Check sheet for the modelled part. Datum: model origin and axes. Units: mm. A direction names the side the tool comes from. Coordinates: 2 decimals unless noted, no trailing zeros. Loops run counter-clockwise (first coordinate to the right, second up) from the corner with the lowest first, then second, coordinate; pieces in that order, holes last.
```python
from build123d import *

# Parameters (mm, degrees)
F0_R     = 5
F1_DEPTH = 12.5
F2_DEPTH = 5
F3_R     = 5
F5_DEPTH = 7.5


with BuildPart() as f1:
    # F0 (on Front) → F1 (new body, symmetric)
    with BuildSketch(Plane.XZ):
        with BuildLine():
            ThreePointArc((6.8596340788, 11.9264922445), (6.9377952197, 12.139972805), (7.0173413473, 12.3529411765))
            ThreePointArc((7.0173413473, 12.3529411765), (6.8474920043, 11.9402854297), (6.6534014969, 11.5384615385))
            ThreePointArc((6.6534014969, 11.5384615385), (6.7556652076, 11.7329300253), (6.8596340788, 11.9264922445))
        make_face()
        with BuildLine():
            ThreePointArc((7.0173413473, -12.3529411765), (6.9377952197, -12.139972805), (6.8596340788, -11.9264922445))
            ThreePointArc((6.8596340788, -11.9264922445), (6.7556652076, -11.7329300253), (6.6534014969, -11.5384615385))
            ThreePointArc((6.6534014969, -11.5384615385), (6.8474920043, -11.9402854297), (7.0173413473, -12.3529411765))
        make_face()
        with BuildLine():
            ThreePointArc((6.6534014969, -11.5384615385), (-3.0597145703, -8.1525079957), (-7.0173413473, -17.6470588235))
            ThreePointArc((-7.0173413473, -17.6470588235), (-6.8474920043, -18.0597145703), (-6.6534014969, -18.4615384615))
            ThreePointArc((-6.6534014969, -18.4615384615), (1.7817812398, -22.2852766326), (7.5, -15))
            ThreePointArc((7.5, -15), (7.3783487348, -13.6546487642), (7.0173413473, -12.3529411765))
            ThreePointArc((7.0173413473, -12.3529411765), (6.8474920043, -11.9402854297), (6.6534014969, -11.5384615385))
        make_face()
        with Locations((0, -15)):
            Circle(F0_R, mode=Mode.SUBTRACT)
        with BuildLine():
            ThreePointArc((6.6534014969, 11.5384615385), (-3.0597145703, 8.1525079957), (-7.0173413473, 17.6470588235))
            ThreePointArc((-7.0173413473, 17.6470588235), (-10.2350656985, 0), (-7.0173413473, -17.6470588235))
            ThreePointArc((-7.0173413473, -17.6470588235), (-3.0597145703, -8.1525079957), (6.6534014969, -11.5384615385))
            ThreePointArc((6.6534014969, -11.5384615385), (6.7556652076, -11.7329300253), (6.8596340788, -11.9264922445))
            ThreePointArc((6.8596340788, -11.9264922445), (4.7649343015, 0), (6.8596340788, 11.9264922445))
            ThreePointArc((6.8596340788, 11.9264922445), (6.7556652076, 11.7329300253), (6.6534014969, 11.5384615385))
        make_face()
        with BuildLine():
            ThreePointArc((7.0173413473, 12.3529411765), (7.3783487348, 13.6546487642), (7.5, 15))
            ThreePointArc((7.5, 15), (1.7817812398, 22.2852766326), (-6.6534014969, 18.4615384615))
            ThreePointArc((-6.6534014969, 18.4615384615), (-6.8474920043, 18.0597145703), (-7.0173413473, 17.6470588235))
            ThreePointArc((-7.0173413473, 17.6470588235), (-3.0597145703, 8.1525079957), (6.6534014969, 11.5384615385))
            ThreePointArc((6.6534014969, 11.5384615385), (6.8474920043, 11.9402854297), (7.0173413473, 12.3529411765))
        make_face()
        with Locations((0, 15)):
            Circle(F0_R, mode=Mode.SUBTRACT)
    extrude(amount=F1_DEPTH, both=True)

    # F0 (on Front) → F2 (join, symmetric)
    with BuildSketch(Plane.XZ):
        with BuildLine():
            ThreePointArc((28.8314064867, -25), (16.0478683636, -21.4844397892), (6.8596340788, -11.9264922445))
            ThreePointArc((6.8596340788, -11.9264922445), (6.9377952197, -12.139972805), (7.0173413473, -12.3529411765))
            ThreePointArc((7.0173413473, -12.3529411765), (7.3783487348, -13.6546487642), (7.5, -15))
            ThreePointArc((7.5, -15), (1.7817812398, -22.2852766326), (-6.6534014969, -18.4615384615))
            ThreePointArc((-6.6534014969, -18.4615384615), (12.7660784434, -36.6320247169), (39.2872644776, -38.6092609833))
            Line((39.2872644776, -38.6092609833), (60, -33))
            Line((60, -33), (48.5096588292, -25))
            Line((48.5096588292, -25), (28.8314064867, -25))
        make_face()
        with BuildLine():
            ThreePointArc((37.2661231393, -28.311901738), (39.719379088, -29.7195718876), (38.3117089384, -32.1728278363))
            Line((38.3117089384, -32.1728278363), (23.8332360697, -36.0937745829))
            ThreePointArc((23.8332360697, -36.0937745829), (21.3799801209, -34.6861044333), (22.7876502706, -32.2328484846))
            Line((22.7876502706, -32.2328484846), (37.2661231393, -28.311901738))
        make_face(mode=Mode.SUBTRACT)
        with BuildLine():
            ThreePointArc((-6.6534014969, 18.4615384615), (1.7817812398, 22.2852766326), (7.5, 15))
            ThreePointArc((7.5, 15), (7.3783487348, 13.6546487642), (7.0173413473, 12.3529411765))
            ThreePointArc((7.0173413473, 12.3529411765), (6.9377952197, 12.139972805), (6.8596340788, 11.9264922445))
            ThreePointArc((6.8596340788, 11.9264922445), (16.0478683636, 21.4844397892), (28.8314064867, 25))
            Line((28.8314064867, 25), (48.5096588292, 25))
            Line((48.5096588292, 25), (60, 33))
            Line((60, 33), (39.2872644776, 38.6092609833))
            ThreePointArc((39.2872644776, 38.6092609833), (12.7660784434, 36.6320247169), (-6.6534014969, 18.4615384615))
        make_face()
        with BuildLine():
            ThreePointArc((22.7876502706, 32.2328484846), (21.3799801209, 34.6861044333), (23.8332360697, 36.0937745829))
            Line((23.8332360697, 36.0937745829), (38.3117089384, 32.1728278363))
            ThreePointArc((38.3117089384, 32.1728278363), (39.719379088, 29.7195718876), (37.2661231393, 28.311901738))
            Line((37.2661231393, 28.311901738), (22.7876502706, 32.2328484846))
        make_face(mode=Mode.SUBTRACT)
    extrude(amount=F2_DEPTH, both=True)

    # F3 (on face) → F5 (cut, symmetric)
    with BuildSketch(Plane(origin=(0, 12.5, 0), x_dir=(-1, 0, 0), z_dir=(0, 1, 0))):
        with Locations((2.7350656985, 0)):
            Circle(F3_R)
    extrude(amount=F5_DEPTH, both=True, mode=Mode.SUBTRACT)


solid = f1.part
```
1) Section check B-B on z = 0. Enter the section's corners in (x, y), plus the area to 3 significant figures.
Answer sheet:
outline: (-10.24, -12.5) - (4.76, -12.5) - (4.76, 12.5) - (2.26, 12.5) - (2.26, 5) - (-7.74, 5) - (-7.74, 12.5) - (-10.24, 12.5) - close
area: 300 mm2
2) Section check A-A on y = -9. Enter the section's corners in (x, z), plus the area to 3 significant figures.
Answer sheet:
outline: (-7.02, -17.65) arc R7.5 ccw to (7.02, -12.35) arc R35 cw to (6.86, -11.93) arc R35 cw to (6.86, 11.93) arc R35 cw to (7.02, 12.35) arc R7.5 ccw to (-7.02, 17.65) arc R50 ccw to start; hole circle Ø10 at (0, -15); hole circle Ø10 at (0, 15)
area: 480 mm2
3) Set-up check for faces 1 (the flat face through (39, 0, 25)), 2 (the flat face through (-3, 5, 0)), 3 (the flat face through (49.789, -0.07, 35.765)): record each of +Z, -Z, +X, -X, +Y, -Y from which the full face is reachable in a straight line by a thin tool's end or side.
Answer sheet:
face 1: +X, +Y, -Y
face 2: +Y
face 3: +Z, +X, +Y, -Y
4) Section check C-C on x = 33.5. Enter the section's corners in (y, z), plus the area to 3 significant figures.
Answer sheet:
outline: (-5, -39.73) - (5, -39.73) - (5, -33.48) - (-5, -33.48) - close; (-5, -29.33) - (5, -29.33) - (5, -25) - (-5, -25) - close; (-5, 25) - (5, 25) - (5, 29.33) - (-5, 29.33) - close; (-5, 33.48) - (5, 33.48) - (5, 39.73) - (-5, 39.73) - close
area: 212 mm2
5) Scan lines: line 1 (Z direction, x = 0, y = -8.5); line 2 (Z direction, x = 0, y = 9.5); line 3 (Z direction, x = 29.5, y = 0.5). Record each from-to range of solid material in increasing order.
Answer sheet:
line 1: z = -22.5 to -20, -10 to 10, 20 to 22.5
line 2: z = -22.5 to -20, -10 to -4.19, 4.19 to 10, 20 to 22.5
line 3: z = -39.99 to -34.56, -30.42 to -25, 25 to 30.42, 34.56 to 39.99
6) Depth check by flat-ended pin: pin 1 (5 mm diameter, centred on x = 36.5, y = -1.5, fed in from +Z); pin 2 (10 mm diameter, centred on y = 4.5, z = 21.5, fed in from +X); pin 3 (5 mm diameter, centred on y = -6.5, z = 6.5, fed in from +X); pin 4 (6 mm diameter, centred on x = 0, z = -15, fed in from -Y). Enter the tip coordinate at first touch or a pass-through.
Answer sheet:
pin 1: stops at z = 39.66
pin 2: stops at x = 50.66
pin 3: stops at x = 5.94
pin 4: passes through
7) Mould release check, pull along X, two halves, no side actions. Record for faces 4 (the cylindrical face through (12.42, 0.07, -36.48)), 5 (the flat face through (54.17, -0.07, 28.94)), 6 (the flat face through (30.97, -0.07, 34.16)), 7 (the flat face through (-1, -12.5, 0)): +X half, -X half, draft (parallel to the pull), parting line (faces both ways), or undercut.
Answer sheet:
face 4: parting line
face 5: +X half
face 6: undercut
face 7: draft
8) Section check D-D on y = -4. Enter the section's corners in (x, z).
Answer sheet:
outline: (-7.02, -17.65) arc R7.5 ccw to (-6.65, -18.46) arc R40 ccw to (39.29, -38.61) - (60, -33) - (48.51, -25) - (28.83, -25) arc R25 cw to (6.86, -11.93) arc R35 cw to (6.86, 11.93) arc R25 cw to (28.83, 25) - (48.51, 25) - (60, 33) - (39.29, 38.61) arc R40 ccw to (-6.65, 18.46) arc R7.5 ccw to (-7.02, 17.65) arc R50 ccw to start; hole circle Ø10 at (0, -15); hole circle Ø10 at (0, 15); hole (22.79, -32.23) arc R2 ccw to (23.83, -36.09) - (38.31, -32.17) arc R2 ccw to (37.27, -28.31) - close; hole (22.79, 32.23) - (37.27, 28.31) arc R2 ccw to (38.31, 32.17) - (23.83, 36.09) arc R2 ccw to start
